Geometry: final body of the model. Coordinates: model frame, mm. A direction names the side the tool comes from. Round coordinates to 2 decimals unless told otherwise and drop trailing zeros. Write each loop counter-clockwise with the first axis right and the second up, starting at its lowest first coordinate (ties: lowest second). Pieces come first, ordered by that corner, then holes. Notation, with made-up numbers: (60.25, 44) - (105.25, 44) arc R23 cw to (105.25, 76) - close; hole circle Ø1 at (20.25, 58). An arc over 180 degrees is marked (long way). Write each question's results on one line, items separated by ' | '.
from build123d import *

# Parameters (mm, degrees)
BLANKSKE_W         = 100
BLANKSKE_H         = 11.75
BLANK_DEPTH        = 12
TOOTHCUTSIM_DEPTH  = 102.400505423
TEETHCUTS_COUNT    = 19
TEETHCUTS_PITCH    = 5.497787138
SKETCH1_R          = 5.1
CUT_EXTRUDE1_DEPTH = 102.400505423


with BuildPart() as part:
    # BlankSke → Blank (new body)
    with BuildSketch(Plane.XY):
        with Locations((50, 5.875)):
            Rectangle(BLANKSKE_W, BLANKSKE_H)
    extrude(amount=-BLANK_DEPTH)

    # TooCutSkeSim → ToothCutSim (cut, through all)
    with BuildSketch(Plane.XY):
        Polygon((0.737261897, 7.8125), (-0.737261897, 7.8125), (-2.179639538, 11.7754), (2.179639538, 11.7754), align=None)
    toothcutsim = extrude(amount=-TOOTHCUTSIM_DEPTH, mode=Mode.SUBTRACT)

    # TeethCuts: ToothCutSim ×19
    with Locations(*[(i * TEETHCUTS_PITCH, 0, 0) for i in range(1, TEETHCUTS_COUNT)]):
        add(toothcutsim, mode=Mode.SUBTRACT)

    # Sketch1 → Cut-Extrude1 (cut, through all)
    with BuildSketch(Plane(origin=(100, 0, 0), x_dir=(0, 0, -1), z_dir=(1, 0, 0))):
        with Locations((6, 0)):
            Circle(SKETCH1_R)
    extrude(amount=-CUT_EXTRUDE1_DEPTH, mode=Mode.SUBTRACT)


solid = part.part
Q1. Section query B-B, the plane y = 10. Give the number of separate pieces and of enclosed holes in the cut face, plus the area to 3 significant figures.
Answer block:
separate pieces: 18 | enclosed holes: 0 | area: 525 mm2
Q2. Ray query, line 1 along Y through (x, z) = (44, -0.5); line 2 along Z through (x, y) = (73, 0.5); line 3 along Y through (x, z) = (17, -4.25). Return the intervals inside material, ascending.
Answer block:
line 1: 0 to 7.81 | line 2: -12 to -11.08, -0.92 to 0 | line 3: 4.79 to 7.81
Q3. Pin query (flat end, axial travel): pin 1 (5 mm diameter, centred on x = 62, z = -8, fed in from -Y); pin 2 (0.7 mm diameter, centred on x = 49.5, z = -5, fed in from +Y); pin 3 (2 mm diameter, centred on y = 2.5, z = -7.5, fed in from +X); pin 4 (1 mm diameter, centred on x = 39.5, z = -5, fed in from -Y). Return the tip coordinate at first contact, or that it passes through.
Answer block:
pin 1: y = 2.4 | pin 2: y = 7.81 | pin 3: through | pin 4: y = 4.87
Q4. Section query A-A, the plane y = 2.25. Return loops of the section in (x, z), plus the area to 3 significant figures.
Answer block:
outline: (0, -12) - (100, -12) - (100, -10.58) - (0, -10.58) - close; (0, -1.42) - (100, -1.42) - (100, 0) - (0, 0) - close | area: 285 mm2
Q5. Mould query, pull axis X, two halves, no side actions, for faces 1 (the flat face through (48.036, 9.754, -5.916)), 2 (the flat face through (1.464, 9.809, -5.916)), 3 (the cylindrical face through (50.7, 5.1, -6.1)), 4 (the flat face through (56.442, 9.809, -5.916)). Classes: pulls with the +X half, pulls with the -X half, needs draft (parallel to the pull), parting line crosses it, or undercut.
Answer block:
face 1: undercut | face 2: pulls with the -X half | face 3: needs draft | face 4: undercut
Q6. Access query for faces 5 (the flat face through (49, 5, 0)), 6 (the flat face through (67.437, 9.809, -5.916)). Directions: +Z, -Z, +X, -X, +Y, -Y. A direction counts if a zero-diameter tool reaches every point of the face in a straight line with its end or side. Return the directions, or none.
Answer block:
face 5: +Z, +X, -X, +Y, -Y | face 6: +Z, -Z, +Y
